```python
from build123d import *

# Parameters (mm, degrees)
BOSS_EXTRUDE1_DEPTH = 2
SKETCH2_R           = 1.5
CUT_EXTRUDE1_DEPTH  = 10
SKETCH3_R           = 1.25
SKETCH3_R_2         = 0.958506699
CUT_EXTRUDE2_DEPTH  = 10
CUT_EXTRUDE3_DEPTH  = 10
SKETCH5_R           = 0.958506699
CUT_EXTRUDE4_DEPTH  = 10
SKETCH8_R           = 2
CUT_EXTRUDE7_DEPTH  = 10
SKETCH9_R           = 5
SKETCH9_R_2         = 2
BOSS_EXTRUDE2_DEPTH = 15
SKETCH11_W          = 20.5
SKETCH11_H          = 25
CUT_EXTRUDE8_DEPTH  = 15
SKETCH12_R          = 1.75
SKETCH12_W          = 35
SKETCH12_H          = 24
CUT_EXTRUDE9_DEPTH  = 15


with BuildPart() as part:
    # Sketch1 → Boss-Extrude1 (new body)
    with BuildSketch(Plane.XY):
        with BuildLine():
            Line((119.800894358, -219.803615077), (119.800894358, -91.803615077))
            ThreePointArc((119.800894358, -91.803615077), (121.922214702, -86.682294733), (116.800894358, -88.803615077))
            Line((116.800894358, -88.803615077), (-21.199105642, -88.803615077))
            ThreePointArc((-21.199105642, -88.803615077), (-26.320425985, -86.682294733), (-24.199105642, -91.803615077))
            Line((-24.199105642, -91.803615077), (-24.199105642, -219.803615077))
            ThreePointArc((-24.199105642, -219.803615077), (-26.320425985, -224.92493542), (-21.199105642, -222.803615077))
            Line((-21.199105642, -222.803615077), (116.800894358, -222.803615077))
            ThreePointArc((116.800894358, -222.803615077), (121.922214702, -224.92493542), (119.800894358, -219.803615077))
        make_face()
    extrude(amount=BOSS_EXTRUDE1_DEPTH)

    # Sketch2 → Cut-Extrude1 (cut)
    with BuildSketch(Plane(origin=(0, 0, 0), x_dir=(-1, 0, 0), z_dir=(0, 0, -1))):
        with Locations((-119.800894358, -88.803615077)):
            Circle(SKETCH2_R)
        with Locations((24.199105642, -88.803615077)):
            Circle(SKETCH2_R)
        with Locations((24.199105642, -222.803615077)):
            Circle(SKETCH2_R)
        with Locations((-119.800894358, -222.803615077)):
            Circle(SKETCH2_R)
    extrude(amount=-CUT_EXTRUDE1_DEPTH, mode=Mode.SUBTRACT)

    # Sketch3 → Cut-Extrude2 (cut)
    with BuildSketch(Plane.XY.offset(2)):
        with Locations((-13.15761234, -148.369936061)):
            Circle(SKETCH3_R)
        with Locations((46.84238766, -148.369936061)):
            Circle(SKETCH3_R)
        with Locations((-13.15761234, -208.369936061)):
            Circle(SKETCH3_R)
        with Locations((46.84238766, -208.369936061)):
            Circle(SKETCH3_R)
        with Locations((46.84238766, -208.369936061)):
            Circle(SKETCH3_R_2, mode=Mode.SUBTRACT)
    extrude(amount=-CUT_EXTRUDE2_DEPTH, mode=Mode.SUBTRACT)

    # Sketch4 → Cut-Extrude3 (cut)
    with BuildSketch(Plane.XY.offset(2)):
        with BuildLine():
            Line((-10.15761234, -149.869936061), (43.84238766, -149.869936061))
            ThreePointArc((43.84238766, -149.869936061), (45.963708003, -150.748615717), (46.84238766, -152.869936061))
            Line((46.84238766, -152.869936061), (46.84238766, -203.869936061))
            ThreePointArc((46.84238766, -203.869936061), (45.963708003, -205.991256404), (43.84238766, -206.869936061))
            Line((43.84238766, -206.869936061), (-10.15761234, -206.869936061))
            ThreePointArc((-10.15761234, -206.869936061), (-12.278932684, -205.991256404), (-13.15761234, -203.869936061))
            Line((-13.15761234, -203.869936061), (-13.15761234, -152.869936061))
            ThreePointArc((-13.15761234, -152.869936061), (-12.278932684, -150.748615717), (-10.15761234, -149.869936061))
        make_face()
    extrude(amount=-CUT_EXTRUDE3_DEPTH, mode=Mode.SUBTRACT)

    # Sketch5 → Cut-Extrude4 (cut)
    with BuildSketch(Plane(origin=(0, 0, 0), x_dir=(-1, 0, 0), z_dir=(0, 0, -1))):
        with Locations((-46.84238766, -208.369936061)):
            Circle(SKETCH5_R)
    extrude(amount=-CUT_EXTRUDE4_DEPTH, mode=Mode.SUBTRACT)

    # Sketch8 → Cut-Extrude7 (cut)
    with BuildSketch(Plane(origin=(0, 0, 0), x_dir=(-1, 0, 0), z_dir=(0, 0, -1))):
        with Locations((-102.369057956, -100.884905857)):
            Circle(SKETCH8_R)
        with Locations((-56.369057956, -100.884905857)):
            Circle(SKETCH8_R)
        with Locations((-102.369057956, -145.884905857)):
            Circle(SKETCH8_R)
        with Locations((-56.369057956, -145.884905857)):
            Circle(SKETCH8_R)
    extrude(amount=-CUT_EXTRUDE7_DEPTH, mode=Mode.SUBTRACT)

    # Sketch9 → Boss-Extrude2 (add)
    with BuildSketch(Plane.XY.offset(2)):
        with Locations((56.369057956, -100.884905857)):
            Circle(SKETCH9_R)
        with Locations((56.369057956, -100.884905857)):
            Circle(SKETCH9_R_2, mode=Mode.SUBTRACT)
        with Locations((102.369057956, -100.884905857)):
            Circle(SKETCH9_R)
        with Locations((102.369057956, -100.884905857)):
            Circle(SKETCH9_R_2, mode=Mode.SUBTRACT)
        with Locations((102.369057956, -145.884905857)):
            Circle(SKETCH9_R)
        with Locations((102.369057956, -145.884905857)):
            Circle(SKETCH9_R_2, mode=Mode.SUBTRACT)
        with Locations((56.369057956, -145.884905857)):
            Circle(SKETCH9_R)
        with Locations((56.369057956, -145.884905857)):
            Circle(SKETCH9_R_2, mode=Mode.SUBTRACT)
    extrude(amount=-BOSS_EXTRUDE2_DEPTH)

    # Sketch11 → Cut-Extrude8 (cut)
    with BuildSketch(Plane.XY.offset(2)):
        with Locations((80.340901452, -178.369936061)):
            Rectangle(SKETCH11_W, SKETCH11_H)
    extrude(amount=-CUT_EXTRUDE8_DEPTH, mode=Mode.SUBTRACT)

    # Sketch12 → Cut-Extrude9 (cut)
    with BuildSketch(Plane.XY.offset(2)):
        with Locations((31.84238766, -106.65983664)):
            Circle(SKETCH12_R)
        with Locations((1.84238766, -106.65983664)):
            Circle(SKETCH12_R)
        with Locations((1.84238766, -134.65983664)):
            Circle(SKETCH12_R)
        with Locations((31.84238766, -134.65983664)):
            Circle(SKETCH12_R)
        with Locations((16.84238766, -120.65983664)):
            Rectangle(SKETCH12_W, SKETCH12_H)
    extrude(amount=-CUT_EXTRUDE9_DEPTH, mode=Mode.SUBTRACT)


solid = part.part
```
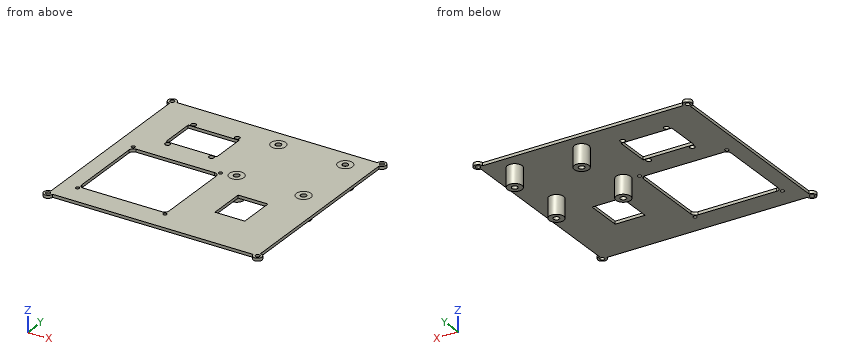
CAD build for the part. Positions are in the model's coordinates, mm. Coordinates: 2 decimals unless noted, no trailing zeros. Write each loop counter-clockwise with the first axis right and the second up, starting at its lowest first coordinate (ties: lowest second). Pieces come first, ordered by that corner, then holes. Notation, with made-up numbers: (5.5, -8) -> (44.5, -8) arc R8 ccw to (44.5, 4) -> close; hole circle Ø11 at (-17, 45.5). An arc over 180 degrees is marked (long way). Return JSON: item names as keys, results as strings. Group by question number.
Q1. Cut at B-B, the plane x = 27. Give the cut face in (y, z), then the cut area to 3 significant figures.
Q2. Drill centre lines: line 1 (Y direction, x = 28, z = 1); line 2 (Y direction, x = 57, z = -5); line 3 (Y direction, x = 1, z = 1). Where is each one in solid material? Low to high.
Q3. Cut at A-A, the plane z = -8. Give the cut face in (x, y), then the cut area to 3 significant figures.
Q4. Flat gauge pins, fed straight in: pin 1 (6 mm diameter, centred on y = -190.5, z = 0, fed in from +X); pin 2 (3 mm diameter, centred on x = 1.84, y = -106.66, fed in from -Z); pin 3 (0.6 mm diameter, centred on x = 20.5, z = 1, fed in from -Y); pin 4 (1.6 mm diameter, centred on y = -122.5, z = 1, fed in from -X). Where does each tip first touch, or does it go through?
Q5. Cut at C-C, the plane y = -173.5. Give the cut face in (x, z), then the cut area to 3 significant figures.
Q6. Cut at D-D, the plane x = 79.5. Give the cut face in (y, z), then the cut area to 3 significant figures.
Returned:
{
 "1": {"outline": "(-222.8, 0) -> (-206.87, 0) -> (-206.87, 2) -> (-222.8, 2) -> close; (-149.87, 0) -> (-132.66, 0) -> (-132.66, 2) -> (-149.87, 2) -> close; (-108.66, 0) -> (-88.8, 0) -> (-88.8, 2) -> (-108.66, 2) -> close", "area": "106 mm2"},
 "2": {"line 1": "y = -222.8 to -206.87, -149.87 to -132.66, -108.66 to -88.8", "line 2": "y = -150.84 to -147.78, -143.99 to -140.92, -105.84 to -102.78, -98.99 to -95.92", "line 3": "y = -222.8 to -206.87, -149.87 to -136.19, -133.13 to -132.66, -108.66 to -108.19, -105.13 to -88.8"},
 "3": {"outline": "circle Ø10 at (56.37, -145.88); circle Ø10 at (56.37, -100.88); circle Ø10 at (102.37, -145.88); circle Ø10 at (102.37, -100.88); hole circle Ø4 at (56.37, -145.88); hole circle Ø4 at (56.37, -100.88); hole circle Ø4 at (102.37, -145.88); hole circle Ø4 at (102.37, -100.88)", "area": "264 mm2"},
 "4": {"pin 1": "stops at x = 119.8", "pin 2": "passes through", "pin 3": "stops at y = -222.8", "pin 4": "stops at x = -24.2"},
 "5": {"outline": "(-24.2, 0) -> (-13.16, 0) -> (-13.16, 2) -> (-24.2, 2) -> close; (46.84, 0) -> (70.09, 0) -> (70.09, 2) -> (46.84, 2) -> close; (90.59, 0) -> (119.8, 0) -> (119.8, 2) -> (90.59, 2) -> close", "area": "127 mm2"},
 "6": {"outline": "(-222.8, 0) -> (-190.87, 0) -> (-190.87, 2) -> (-222.8, 2) -> close; (-165.87, 0) -> (-88.8, 0) -> (-88.8, 2) -> (-165.87, 2) -> close", "area": "218 mm2"}
}
